from build123d import *

# Parameters (mm, degrees)
SKETCH_R        = 25
PAD_DEPTH       = 25
PAD_TAPER       = 15
SKETCH001_R     = 21.044581
POCKET_DEPTH    = 17
POCKET_TAPER    = 15
SKETCH002_R     = 14.009915
PAD001_DEPTH    = 30
PAD001_TAPER    = 20
SKETCH003_R     = 2.189118
POCKET001_DEPTH = 20


with BuildPart() as part:
    # Sketch → Pad (new body)
    with BuildSketch(Plane.XY):
        Circle(SKETCH_R)
    extrude(amount=PAD_DEPTH, taper=PAD_TAPER)

    # Sketch001 (on Face2 of Pad) → Pocket (cut)
    with BuildSketch(Plane(origin=(0, 0, 0), x_dir=(1, 0, 0), z_dir=(0, 0, -1))):
        Circle(SKETCH001_R)
    extrude(amount=-POCKET_DEPTH, taper=POCKET_TAPER, mode=Mode.SUBTRACT)

    # Sketch002 (on Face5 of Pocket) → Pad001 (join)
    with BuildSketch(Plane(origin=(0, 0, 17), x_dir=(1, 0, 0), z_dir=(0, 0, -1))):
        Circle(SKETCH002_R)
    extrude(amount=PAD001_DEPTH, taper=PAD001_TAPER)

    # Sketch003 (on Face7 of Pad001) → Pocket001 (cut)
    with BuildSketch(Plane(origin=(0, 0, -13), x_dir=(1, 0, 0), z_dir=(0, 0, -1))):
        Circle(SKETCH003_R)
    extrude(amount=-POCKET001_DEPTH, mode=Mode.SUBTRACT)


solid = part.part
Design review of the part built by this model. Coordinates are the model's own, in mm. A direction names the side the tool comes from. Coordinates: 2 decimals unless noted, no trailing zeros. Loops run counter-clockwise (first coordinate to the right, second up) from the corner with the lowest first, then second, coordinate; pieces in that order, holes last. Notation, with made-up numbers: (71.5, -8.5) - (96.5, -8.5) arc R20 cw to (96.5, 3.5) - close; hole circle Ø11 at (73, -29.75). An arc over 180 degrees is marked (long way). Use CSV: the item, a comma, the result in double quotes. Start each with the question number.
1. Add section D-D on z = 12. Give the boundary of the cut face in (x, y).
2. Add section A-A on x = 0. Give the boundary of the cut face in (y, z).
3. Mouldability with a two-part tool opening along X and no side actions: class faces 1 (the flat face through (0, 0, 25)), 2 (the conical face through (9.282, -17.846, 18.231)), 3 (the flat face through (0, 0, 7)) as released by +X, released by -X, zero draft, split by the parting line, or undercut.
4. Clearance check with flat-ended pins moving along their axes: pin 1 (4 mm diameter, centred on x = 0, y = 0, fed in from -Z); pin 2 (2 mm diameter, centred on y = -18, z = 7, fed in from +X); pin 3 (4 mm diameter, centred on x = -18, z = 17, fed in from +Y). State where each tip first meets the part, or that it passes through.
5. Add section B-B on z = 16. Give the boundary of the cut face in (x, y).
6. For faces 4 (the flat face through (1.3, 2, -13)), 5 (the cylindrical face through (-1.74, 1.33, -3.14)), list the 3-axis set-ups (+Z, -Z, +X, -X, +Y, -Y) from which the entire face can be reached by the end or side of a thin tool; tool diameter is ignored.
7. Add section C-C on z = -3.5. Give the boundary of the cut face in (x, y), plus the area to 3 significant figures.
8. To check wall thickness, follow probe 1 along Y at (x, z) = (-3, 13); probe 2 along X at (y, z) = (-4.5, 11); probe 3 along Y at (x, z) = (0, 2). State the ranges of each line that lie inside material, in increasing order.
Resolved:
1,outline,"circle Ø43.57 at (0, 0); circle Ø24.38 at (0, 0); hole circle Ø35.66 at (0, 0)"
2,outline,"(-25, 0) - (-21.04, 0) - (-16.49, 17) - (-14.01, 17) - (-3.09, -13) - (-2.19, -13) - (-2.19, 7) - (2.19, 7) - (2.19, -13) - (3.09, -13) - (14.01, 17) - (16.49, 17) - (21.04, 0) - (25, 0) - (18.3, 25) - (-18.3, 25) - close"
3,face 1,"zero draft"
3,face 2,"split by the parting line"
3,face 3,"undercut"
4,pin 1,"z = 7"
4,pin 2,"x = 15.75"
4,pin 3,"y = 12.87"
5,outline,"circle Ø41.43 at (0, 0); circle Ø27.29 at (0, 0); hole circle Ø33.51 at (0, 0)"
6,face 4,"-Z, +X, -X, +Y, -Y"
6,face 5,"-Z"
7,outline,"circle Ø13.1 at (0, 0); hole circle Ø4.38 at (0, 0)"
7,area,"120 mm2"
8,probe 1,"-21.31 to -17.3, -12.19 to 12.19, 17.3 to 21.31"
8,probe 2,"-21.59 to -17.53, -10.94 to 10.94, 17.53 to 21.59"
8,probe 3,"-24.46 to -20.51, -8.55 to -2.19, 2.19 to 8.55, 20.51 to 24.46"
